```python
from build123d import *

# Parameters (mm, degrees)
ESBO_O1_R                  = 4
ESBO_O1_W                  = 13
ESBO_O1_H                  = 16
RESSALTO_EXTRUS_O1_DEPTH   = 14
RESSALTO_EXTRUS_O2_START   = -4
ESBO_O3_R                  = 8
ESBO_O3_R_2                = 1.5
RESSALTO_EXTRUS_O2_DEPTH   = 4
CORTE_EXTRUS_O1_DEPTH      = 71.215738976
CORTE_EXTRUS_O1_DEPTH_BACK = 71.215738976
ESBO_O2_R                  = 1.6
CORTE_EXTRUS_O2_START      = 2
CORTE_EXTRUS_O2_DEPTH      = 2
FILETE1_R                  = 2.5


with BuildPart() as part:
    # Esboço1 → Ressalto-extrusão1 (new body)
    with BuildSketch(Plane.XY):
        with BuildLine():
            Line((2.5, 52.400657923), (2.5, 41))
            Line((2.5, 41), (8, 41))
            Line((8, 41), (8, 19))
            Line((8, 19), (2.5, 19))
            Line((2.5, 19), (2.5, 7.599342077))
            ThreePointArc((2.5, 7.599342077), (0, -8), (-2.5, 7.599342077))
            Line((-2.5, 7.599342077), (-2.5, 19))
            Line((-2.5, 19), (-13, 19))
            Line((-13, 19), (-13, 41))
            Line((-13, 41), (-2.5, 41))
            Line((-2.5, 41), (-2.5, 52.400657923))
            ThreePointArc((-2.5, 52.400657923), (0, 68), (2.5, 52.400657923))
        make_face()
        with Locations((0, 60)):
            Circle(ESBO_O1_R, mode=Mode.SUBTRACT)
        Circle(ESBO_O1_R, mode=Mode.SUBTRACT)
        with Locations((-2.5, 30)):
            Rectangle(ESBO_O1_W, ESBO_O1_H, mode=Mode.SUBTRACT)
    extrude(amount=RESSALTO_EXTRUS_O1_DEPTH)

    # Esboço3 → Ressalto-extrusão2 (add)
    # profile 1 of 2: a face of its own
    with BuildSketch(Plane.XY.offset(14).offset(RESSALTO_EXTRUS_O2_START)):
        with Locations((0, 60)):
            Circle(ESBO_O3_R)
        with Locations((0, 60)):
            Circle(ESBO_O3_R_2, mode=Mode.SUBTRACT)
    # profile 2 of 2: a face of its own
    with BuildSketch(Plane.XY.offset(14).offset(RESSALTO_EXTRUS_O2_START)):
        Circle(ESBO_O3_R)
        Circle(ESBO_O3_R_2, mode=Mode.SUBTRACT)
    extrude(amount=RESSALTO_EXTRUS_O2_DEPTH)

    # Esboço2 → Corte-extrusão1 (cut, two sides: drawn at the far end of the back side and taken through both)
    with BuildSketch(Plane.ZY.offset(2.5).offset(-CORTE_EXTRUS_O1_DEPTH_BACK)):
        with Locations(Location((7, 30, 0), (0, 0, 270))):
            Circle(ESBO_O2_R)
    extrude(amount=CORTE_EXTRUS_O1_DEPTH + CORTE_EXTRUS_O1_DEPTH_BACK, mode=Mode.SUBTRACT)

    # Esboço4 → Corte-extrusão2 (cut)
    with BuildSketch(Plane.XY.offset(10).offset(CORTE_EXTRUS_O2_START)):
        Polygon((0, 56.940043573), (2.65, 58.470021787), (2.65, 61.529978213), (0, 63.059956427), (-2.65, 61.529978213), (-2.65, 58.470021787), align=None)
        Polygon((0, -3.059956427), (2.65, -1.529978213), (2.65, 1.529978213), (0, 3.059956427), (-2.65, 1.529978213), (-2.65, -1.529978213), align=None)
    extrude(amount=-CORTE_EXTRUS_O2_DEPTH, mode=Mode.SUBTRACT)

    # Filete1
    filete1_edges = [part.edges().sort_by_distance(p)[0] for p in [
        (-2.5, 19, 7),
        (-13, 19, 7),
        (-13, 41, 7),
        (-2.5, 41, 7),
        (2.5, 41, 7),
        (8, 41, 7),
        (8, 19, 7),
        (2.5, 19, 7),
    ]]
    fillet(filete1_edges, radius=FILETE1_R)


solid = part.part
```
The model under review builds one solid part; all positions refer to its coordinate system, in mm. A direction names the side the tool comes from. Coordinates: 2 decimals unless noted, no trailing zeros. Write each loop counter-clockwise with the first axis right and the second up, starting at its lowest first coordinate (ties: lowest second). Pieces come first, ordered by that corner, then holes. Notation, with made-up numbers: (-10, -10) -> (-4, -10) arc R27 cw to (-4, 11) -> close; hole circle Ø3 at (-12.5, 89). An arc over 180 degrees is marked (long way). One line per item, written item: value. Start each with the question number.
Q1. Add section C-C, the plane z = 13. Give the boundary of the cut face in (x, y).
Q2. The part is to be moulded in two halves that separate along Y. For faces 1 (the face through (5, 31, 0)), 2 (the face through (6.03, 31.27, 6.03)), say which applies: +Y half, -Y half, draft (parallel to the pull), parting line (faces both ways), or undercut.
Q3. Add section D-D, the plane x = -6.5. Give the boundary of the cut face in (y, z), then the cut area to 3 significant figures.
Q4. Clearance check with flat-ended pins moving along their axes: P1, Ø6, axis at x = -7, z = 5, coming from the -Y side; P2, Ø5, axis at y = 51.5, z = 5.5, coming from the -X side; P3, Ø4.5, axis at y = 49.5, z = 10, coming from the -X side; P4, Ø2.5, axis at x = 0, y = 0, coming from the +Z side. State where each tip first meets the part, or that it passes through.
Q5. Add section A-A, the plane z = 7. Count the separate pieces of the cut face and the enclosed holes in it, then the cut area to 3 significant figures.
Q6. To check wall thickness, follow probe 1 along Y at (x, z) = (0, 3.25); probe 2 along X at (y, z) = (28.5, 5); probe 3 along Y at (x, z) = (0, 13.1). State the ranges of each line that lie inside material, in increasing order.
Q7. Add section B-B, the plane y = 30. Give the boundary of the cut face in (x, z).
Q8. For faces 3 (the face through (-3, 42, 7)), 4 (the face through (-3, 22, 7)), 5 (the face through (2.65, 60, 11)), list the 3-axis set-ups (+Z, -Z, +X, -X, +Y, -Y) from which the entire face can be reached by the end or side of a thin tool; tool diameter is ignored.
Response:
1. outline: (-13, 21.5) arc R2.5 ccw to (-10.5, 19) -> (-5, 19) arc R2.5 cw to (-2.5, 16.5) -> (-2.5, 7.6) arc R8 ccw (long way) to (2.5, 7.6) -> (2.5, 16.5) arc R2.5 cw to (5, 19) -> (5.5, 19) arc R2.5 ccw to (8, 21.5) -> (8, 38.5) arc R2.5 ccw to (5.5, 41) -> (5, 41) arc R2.5 cw to (2.5, 43.5) -> (2.5, 52.4) arc R8 ccw (long way) to (-2.5, 52.4) -> (-2.5, 43.5) arc R2.5 cw to (-5, 41) -> (-10.5, 41) arc R2.5 ccw to (-13, 38.5) -> close; hole (-9, 22) -> (4, 22) -> (4, 38) -> (-9, 38) -> close; hole circle Ø3 at (0, 0); hole circle Ø3 at (0, 60)
2. face 1: draft
2. face 2: undercut
3. outline: (-4.66, 0) -> (4.66, 0) -> (4.66, 14) -> (-4.66, 14) -> close; (19, 0) -> (22, 0) -> (22, 14) -> (19, 14) -> close; (38, 0) -> (41, 0) -> (41, 14) -> (38, 14) -> close; (55.34, 0) -> (64.66, 0) -> (64.66, 14) -> (55.34, 14) -> close
3. area: 345 mm²
4. P1: y = -6.93
4. P2: x = -5.29
4. P3: x = -2.5
4. P4: through
5. separate pieces: 2
5. enclosed holes: 2
5. area: 641 mm²
6. probe 1: -8 to -4, 4 to 22, 38 to 56, 64 to 68
6. probe 2: -13 to -9, 4 to 8
6. probe 3: -8 to -1.5, 1.5 to 22, 38 to 58.5, 61.5 to 68
7. outline: (-13, 0) -> (-9, 0) -> (-9, 5.4) -> (-13, 5.4) -> close; (-13, 8.6) -> (-9, 8.6) -> (-9, 14) -> (-13, 14) -> close; (4, 0) -> (8, 0) -> (8, 5.4) -> (4, 5.4) -> close; (4, 8.6) -> (8, 8.6) -> (8, 14) -> (4, 14) -> close
8. face 3: +Z, -Z, -X
8. face 4: +Z, -Z
8. face 5: -Z
